from build123d import *

# Parameters (mm, degrees)
SKETCH1_W               = 20
SKETCH1_H               = 16.9
BOSS_EXTRUDE1_DEPTH     = 23.75
SKETCH2_R               = 8.45
BOSS_EXTRUDE2_DEPTH     = 236
SKETCH6_R               = 18.45
SKETCH6_R_2             = 8.45
CUT_EXTRUDE_THIN1_DEPTH = 30
CUT_EXTRUDE1_START      = 5
SKETCH7_W               = 150
SKETCH7_H               = 40
CUT_EXTRUDE1_DEPTH      = 10


with BuildPart() as part:
    # Sketch1 → Boss-Extrude1 (new, symmetric)
    with BuildSketch(Plane(origin=(0, 0, 0), x_dir=(0, 0, -1), z_dir=(1, 0, 0))):
        Rectangle(SKETCH1_W, SKETCH1_H)
    extrude(amount=BOSS_EXTRUDE1_DEPTH, both=True)

    # Sketch2 → Boss-Extrude2 (add)
    with BuildSketch(Plane(origin=(23.75, 0, 0), x_dir=(0, 0, -1), z_dir=(1, 0, 0))):
        with Locations(Location((0, 0, 0), (0, 0, 270))):
            Circle(SKETCH2_R)
    boss_extrude2 = extrude(amount=BOSS_EXTRUDE2_DEPTH)

    # Sketch3 → M10x1.25 Tapped Hole1 (revolve, cut)
    with BuildSketch(Plane(origin=(259.75, 0, 0), x_dir=(0, 0, -1), z_dir=(0, 1, 0))):
        Polygon((0, 0), (0, 32.643786724), (4.4, 30), (4.4, 0), align=None)
    m10x1_25_tapped_hole1 = revolve(axis=Axis((266.1, 0, 0), (-1, 0, 0)), mode=Mode.SUBTRACT)

    # Mirror1: Boss-Extrude2, M10x1.25 Tapped Hole1 across plane
    add(boss_extrude2.mirror(Plane(origin=(0, 0, 0), x_dir=(0, 0, 1), z_dir=(1, 0, 0))))
    add(m10x1_25_tapped_hole1.mirror(Plane(origin=(0, 0, 0), x_dir=(0, 0, 1), z_dir=(1, 0, 0))), mode=Mode.SUBTRACT)

    # Sketch6 → Cut-Extrude-Thin1 (cut, symmetric)
    with BuildSketch(Plane(origin=(0, 0, 0), x_dir=(0, 0, -1), z_dir=(1, 0, 0))):
        Circle(SKETCH6_R)
        Circle(SKETCH6_R_2, mode=Mode.SUBTRACT)
    extrude(amount=CUT_EXTRUDE_THIN1_DEPTH, both=True, mode=Mode.SUBTRACT)

    # Sketch7 → Cut-Extrude1 (cut)
    with BuildSketch(Plane(origin=(0, 0, 0), x_dir=(1, 0, 0), z_dir=(0, 1, 0)).offset(CUT_EXTRUDE1_START)):
        Rectangle(SKETCH7_W, SKETCH7_H)
    extrude(amount=CUT_EXTRUDE1_DEPTH, mode=Mode.SUBTRACT)


solid = part.part
Geometry: final body of the model. Coordinates: model frame, mm. A direction names the side the tool comes from. Give positions to 0.01 mm unless a question says otherwise; leave off trailing zeros. Loops run counter-clockwise (first coordinate to the right, second up) from the corner with the lowest first, then second, coordinate; pieces in that order, holes last. Notation, with made-up numbers: (-35.75, 8) -> (10.25, 8) arc R23 ccw to (10.25, 32) -> close; hole circle Ø11 at (0.5, 57). An arc over 180 degrees is marked (long way). Put each result on its own line as item: value.
1. Pull-direction query (X, two-part tool) for faces 3 (the flat face through (-1, 5, 0)), 4 (the cylindrical face through (-244.96, -1.322, -4.197)), 5 (the conical face through (227.565, 0.465, 0.606)), 6 (the conical face through (-227.565, 0.465, 0.606)); classes: released by +X, released by -X, zero draft, split by the parting line, or undercut.
Taken from the geometry:
face 3: undercut
face 4: zero draft
face 5: released by +X
face 6: released by -X
2. Set-up query: faces 1 (the flat face through (259.75, -4, 4)), 2 (the cylindrical face through (244.96, -1.322, -4.197)). Return all of +Z, -Z, +X, -X, +Y, -Y with unobstructed straight access to the full face (end or side cutting, diameter ignored); none if empty.
Taken from the geometry:
face 1: +Z, -Z, +X, +Y, -Y
face 2: +X
3. Pin query (flat end, axial travel): P1, Ø1.5, axis at y = 0.5, z = 0, coming from the -X side; P2, Ø6, axis at x = 158.5, y = 6, coming from the +Z side; P3, Ø3, axis at x = -165.5, y = -4, coming from the -Z side. Return the tip coordinate at first contact, or that it passes through.
Taken from the geometry:
P1: stops at x = -227.86
P2: stops at z = 7.9
P3: stops at z = -8.07
4. Cut plane B-B (x = 199.5). Return the cut outline in (y, z), plus the area to 3 significant figures.
Taken from the geometry:
outline: circle Ø16.9 at (0, 0)
area: 224 mm2
5. Ray query, line 1 along X through (y, z) = (6.5, 2.5); line 2 along Z through (x, y) = (-237, 0). Return the intervals inside material, ascending. Write a range as [from, to].
Taken from the geometry:
line 1: x = [-259.75, -75], [75, 259.75]
line 2: z = [-8.45, -4.4], [4.4, 8.45]
6. Cut plane A-A (x = -68.5). Return the cut outline in (y, z), plus the area to 3 significant figures.
Taken from the geometry:
outline: (5, -6.81) -> (5, 6.81) arc R8.45 ccw (long way) to start
area: 191 mm2
